Verification items for the finished model (mm, model axes). A direction names the side the tool comes from. Give positions to 0.01 mm unless a question says otherwise; leave off trailing zeros. Loops run counter-clockwise (first coordinate to the right, second up) from the corner with the lowest first, then second, coordinate; pieces in that order, holes last. Notation, with made-up numbers: M 48.5,61.25 L 85.5,61.25 A29 ccw 85.5,85.25 Z; hole C 24.25,-13.75 d6. An arc over 180 degrees is marked long. Use a Markdown table: item, result.
from build123d import *

# Parameters (mm, degrees)
F0_R     = 15.875
F1_DEPTH = 50.8
F2_DEPTH = 25.4
F0_R_2   = 9.525
F3_DEPTH = 12.7
F4_R     = 6.35
F4_R_2   = 6.3499


# Not quite as in the source:
# - a fillet or chamfer is up to 0.001 mm smaller than in the source, because OpenCascade refuses the exact size


with BuildPart() as f1:
    # F0 (on Top) → F1 (new body)
    with BuildSketch(Plane.XY):
        with BuildLine():
            ThreePointArc((-21.53046875, -28.0682110263), (-4.8697649831, -18.2130603251), (1.68671875, 0))
            ThreePointArc((1.68671875, 0), (-4.8697649831, 18.2130603251), (-21.53046875, 28.0682110263))
            ThreePointArc((-21.53046875, 28.0682110263), (-55.46328125, 0), (-21.53046875, -28.0682110263))
        make_face()
        with Locations((-26.88828125, 0)):
            Circle(F0_R, mode=Mode.SUBTRACT)
    extrude(amount=F1_DEPTH)

    # F0 (on Top) → F2 (join)
    with BuildSketch(Plane.XY):
        with BuildLine():
            ThreePointArc((-21.53046875, 28.0682110263), (-4.8697649831, 18.2130603251), (1.68671875, 0))
            ThreePointArc((1.68671875, 0), (-4.8697649831, -18.2130603251), (-21.53046875, -28.0682110263))
            Line((-21.53046875, -28.0682110263), (27.48359375, -18.7121406842))
            ThreePointArc((27.48359375, -18.7121406842), (4.86171875, 0), (27.48359375, 18.7121406842))
            Line((27.48359375, 18.7121406842), (-21.53046875, 28.0682110263))
        make_face()
    extrude(amount=F2_DEPTH)

    # F0 (on Top) → F3 (join)
    with BuildSketch(Plane.XY):
        with BuildLine():
            ThreePointArc((42.96171875, 0), (38.5907295946, 12.1420402167), (27.48359375, 18.7121406842))
            ThreePointArc((27.48359375, 18.7121406842), (4.86171875, 0), (27.48359375, -18.7121406842))
            ThreePointArc((27.48359375, -18.7121406842), (38.5907295946, -12.1420402167), (42.96171875, 0))
        make_face()
        with Locations((23.91171875, 0)):
            Circle(F0_R_2, mode=Mode.SUBTRACT)
    extrude(amount=F3_DEPTH)

    # F4 (call 1 of 2: OpenCascade refuses the feature's edges together)
    f4_edges = [f1.edges().sort_by_distance(p)[0] for p in [
        (27.483594, -18.712141, 6.35),
        (27.483594, -18.712141, 19.05),
    ]]
    fillet(f4_edges, radius=F4_R)

    # F4#2 (call 2 of 2) (radius 6.35 in the source; OpenCascade refuses exactly that, so slightly less here)
    f4_2_edges = [f1.edges().sort_by_distance(p)[0] for p in [
        (27.483594, 18.712141, 6.35),
        (27.483594, 18.712141, 19.05),
    ]]
    fillet(f4_2_edges, radius=F4_R_2)


solid = f1.part
(1) Cross-section at C-C on y = 1. Record the cut outline in (x, z), then the cut area to 3 significant figures.
Results below:
| item | result |
|---|---|
| outline | M -55.45,0 L -42.73,0 L -42.73,50.8 L -55.45,50.8 Z; M -11.04,0 L 14.44,0 L 14.44,12.7 L 4.89,12.7 L 4.89,25.4 L 1.67,25.4 L 1.67,50.8 L -11.04,50.8 Z; M 33.38,0 L 42.94,0 L 42.94,12.7 L 33.38,12.7 Z |
| area | 1,620 mm^2 |
(2) Gauge pin test, flat ends, axial feed: P1, Ø6, axis at x = 4.5, z = 18, coming from the +Y side; P2, Ø8, axis at x = 20, y = -11, coming from the +Z side; P3, Ø5, axis at y = 9, z = 6.5, coming from the +X side. Record the tip position at first contact, or that the pin passes through.
Results below:
| item | result |
|---|---|
| P1 | y = 23.67 |
| P2 | z = 12.7 |
| P3 | x = 41.82 |
(3) Material ranges on line 1 (Z direction, x = 3, y = -23); line 2 (X direction, y = 4.5, z = 10); line 3 (Z direction, x = 13.5, y = -11.5), recorded low to high.
Results below:
| item | result |
|---|---|
| line 1 | 0 to 25.4 |
| line 2 | -55.11 to -42.11, -11.66 to 15.52, 32.31 to 42.42 |
| line 3 | 0 to 12.7 |
(4) Cross-section at A-A on z = 11.5. Record the cut outline in (x, y) (3 decimals).
Results below:
| item | result |
|---|---|
| outline | M -21.53,-28.068 L 27.484,-18.712 A19.05 ccw 27.484,18.712 L -21.53,28.068 A28.575 ccw long Z; hole C -26.888,0 d31.75; hole C 23.912,0 d19.05 |
(5) Cross-section at B-B on x = 30. Record the cut outline in (y, z).
Results below:
| item | result |
|---|---|
| outline | M -18.05,0 L -7.33,0 L -7.33,12.7 L -18.05,12.7 Z; M 7.33,0 L 18.05,0 L 18.05,12.7 L 7.33,12.7 Z |
(6) Draft check along X on faces 3 (the cylindrical face through (14.396, 0.419, 6.261)), 4 (the flat face through (-2.813, -24.495, 9.7)), 5 (the flat face through (15, -5, 12.7)). Enter one of: +X half, -X half, draft (parallel to the pull), parting line (faces both ways), or undercut.
Results below:
| item | result |
|---|---|
| face 3 | undercut |
| face 4 | +X half |
| face 5 | draft |
(7) Set-up check for faces 1 (the cylindrical face through (10.652, -18.774, 19.139)), 2 (the flat face through (-15, -12, 50.8)): record each of +Z, -Z, +X, -X, +Y, -Y from which the full face is reachable in a straight line by a thin tool's end or side.
Results below:
| item | result |
|---|---|
| face 1 | +Z, +X |
| face 2 | +Z, +X, -X, +Y, -Y |
(8) Cross-section at D-D on x = -9. Record the cut outline in (y, z).
Results below:
| item | result |
|---|---|
| outline | M -25.68,0 L 25.68,0 L 25.68,25.4 L 22.28,25.4 L 22.28,50.8 L -22.28,50.8 L -22.28,25.4 L -25.68,25.4 Z |
